CAD build for the part. Positions are in the model's coordinates, mm. A direction names the side the tool comes from. Round coordinates to 2 decimals unless told otherwise and drop trailing zeros. Write each loop counter-clockwise with the first axis right and the second up, starting at its lowest first coordinate (ties: lowest second). Pieces come first, ordered by that corner, then holes. Notation, with made-up numbers: (83.5, 16.25) - (97.5, 16.25) arc R30 ccw to (97.5, 46.25) - close; hole circle Ø1 at (49, 41.5). An arc over 180 degrees is marked (long way). Use one line per item in the form item = value. Start each with the question number.
Item 1: Band-saw the part on A-A, the plane x = 0. List the corners of the cut face in (y, z), and give its area (3 significant figures).
Item 2: Band-saw the part on B-B, the plane z = 0. List the corners of the cut face in (x, y), and give its area (3 significant figures).
Item 3: Band-saw the part on C-C, the plane y = 0.85. List the corners of the cut face in (x, z).
Item 4: Tool access for faces 5 (the flat face through (-2.8, -1.751, -9.3)), 6 (the cylindrical face through (5.77, -1.16, -7.53)), 7 (the flat face through (4, -1.151, 11)): list every direction of +Z, -Z, +X, -X, +Y, -Y with a clear straight run to the whole face (end or side of a thin tool).
Item 5: Pin check, flat tips, straight feed: pin 1 (1.5 mm diameter, centred on x = -3, z = -3, fed in from +Y); pin 2 (5 mm diameter, centred on x = -1, z = 0, fed in from -Y). Stop position of each tip, or through.
Item 6: Drill centre lines: L1, parallel to X at y = -1.35, z = 0; L2, parallel to Z at x = -2.5, y = 0.15. Where is each one in solid material? Low to high.
Item 7: Pull direction X, two halves, no side cores. Call faces 1 (the flat face through (0, -0.051, 0)), 2 (the flat face through (0, -0.751, 0)), 3 (the flat face through (8, 1.449, -1)), 4 (the conical face through (8.04, 1.29, 4.18)): +X half, -X half, draft (parallel to the pull), parting line (faces both ways), or undercut.
Autodesk Inventor part; units mm, degrees
ref_plane "YZ Plane" through (0, 0, 0) normal (1, 0, 0) x (0, 1, 0)
ref_plane "XZ Plane" through (0, 0, 0) normal (0, 1, 0) x (-1, 0, 0)
ref_plane "XY Plane" through (0, 0, 0) normal (0, 0, 1) x (1, 0, 0)
sketch "Skizze1" plane through (0, 0, 0) normal (1, 0, 0) x (0, 1, 0)
  line L0 (3, 8.0893) -> (5.1212, 8.0893) construction
  line L1 (-0.0509, -6.2) -> (0.0741, -6.2) construction
  line L2 (0.0741, -6.2) -> (0.0741, 6.2) construction
  line L3 (0.0741, 6.2) -> (-0.0509, 6.2) construction
  line L4 (-0.0509, 6.2) -> (-0.0509, -6.2) construction
  line L5 (-0.0509, -6.2) -> (0.0741, 6.2) construction
  line L6 (0.0741, -6.2) -> (-0.0509, 6.2) construction
  line L7 (-0.0509, 6.2) -> (-0.0509, 0)
  line L8 (-0.0509, 0) -> (-0.7509, 0)
  line L9 (-0.7509, 0) -> (-0.7509, 7.0138)
  line L10 (-0.7509, 7.0138) -> (0.4491, 8.2138)
  line L11 (0.4491, 8.2138) -> (0.4491, 8.4858)
  line L12 (-0.0509, 6.2) -> (-0.0509, 6.4)
  line L13 (-0.0509, 6.4) -> (1.4491, 7.9)
  line L14 (1.4491, 7.9) -> (1.4491, 8.9)
  line L15 (1.4491, 8.9) -> (-1.1509, 11.5)
  line L16 (-1.7509, 12.5) -> (-1.7509, 9.4858)
  line L17 (0.4491, 8.4858) -> (-0.5509, 9.4858)
  line L18 (-0.5509, 9.4858) -> (-1.7509, 9.4858)
  line L19 (-1.1509, 11.5) -> (-1.1509, 12.5)
  line L20 (-1.1509, 12.5) -> (-1.7509, 12.5)
  line L21 (1.4491, 8.9) -> (1.4491, -8.9)
  line L22 (-1.1509, 11.5) -> (1.4491, 8.9)
  line L23 (1.4491, 7.9) -> (0.1491, 6.6)
  point P0 (0.0116, 0)
  point P1 (0.0116, 0)
  dimension "d14" = 0.125
  dimension "d16" = 0.7
  dimension "d18" = 135
  dimension "d20" = 0.2
  dimension "d27" = 135
  dimension "d28" = 1
  dimension "d29" = 1.2
  dimension "d30" = 1
  dimension "d31" = 1
  dimension "d34" = 1
  dimension "d36" = 0.6
  dimension "d37" = 12.5
  dimension "d39" = 1
revolve "Umdrehung1" add sketch "Skizze1" angle 360 about axis through (0, -0.0509, 0) along (0, -1, 0)
properties part number "50_ETL_Membrane_v0"
Determined:
q1.outline = (-1.75, -12.5) - (-1.15, -12.5) - (-1.15, -11.5) - (1.45, -8.9) - (1.45, -7.9) - (-0.05, -6.4) - (-0.05, 6.4) - (1.45, 7.9) - (1.45, 8.9) - (-1.15, 11.5) - (-1.15, 12.5) - (-1.75, 12.5) - (-1.75, 9.49) - (-0.55, 9.49) - (0.45, 8.49) - (0.45, 8.21) - (-0.75, 7.01) - (-0.75, -7.01) - (0.45, -8.21) - (0.45, -8.49) - (-0.55, -9.49) - (-1.75, -9.49) - close
q1.area = 24.1 mm²
q2.outline = (-12.5, -1.75) - (-9.49, -1.75) - (-9.49, -0.55) - (-8.49, 0.45) - (-8.21, 0.45) - (-7.01, -0.75) - (7.01, -0.75) - (8.21, 0.45) - (8.49, 0.45) - (9.49, -0.55) - (9.49, -1.75) - (12.5, -1.75) - (12.5, -1.15) - (11.5, -1.15) - (8.9, 1.45) - (7.9, 1.45) - (6.4, -0.05) - (-6.4, -0.05) - (-7.9, 1.45) - (-8.9, 1.45) - (-11.5, -1.15) - (-12.5, -1.15) - close
q2.area = 24.1 mm²
q3.outline = circle Ø19 at (0, 0); hole circle Ø14.6 at (0, 0)
q4.face_5 = +Z, -Z, +X, -X, -Y
q4.face_6 = -Y
q4.face_7 = +Y
q5.pin_1 = -0.05
q5.pin_2 = -0.75
q6.L1 = -12.5 to -9.49, 9.49 to 12.5
q6.L2 = -9.89 to -8.42, -7.51 to -6.11, 6.11 to 7.51, 8.42 to 9.89
q7.face_1 = undercut
q7.face_2 = undercut
q7.face_3 = draft
q7.face_4 = parting line
